Drawing for the job (mm, zero at the part's lowest x, y, z). Coordinates: 2 decimals unless noted, no trailing zeros. Write each loop counter-clockwise with the first axis right and the second up, starting at its lowest first coordinate (ties: lowest second). Pieces come first, ordered by that corner, then holes.
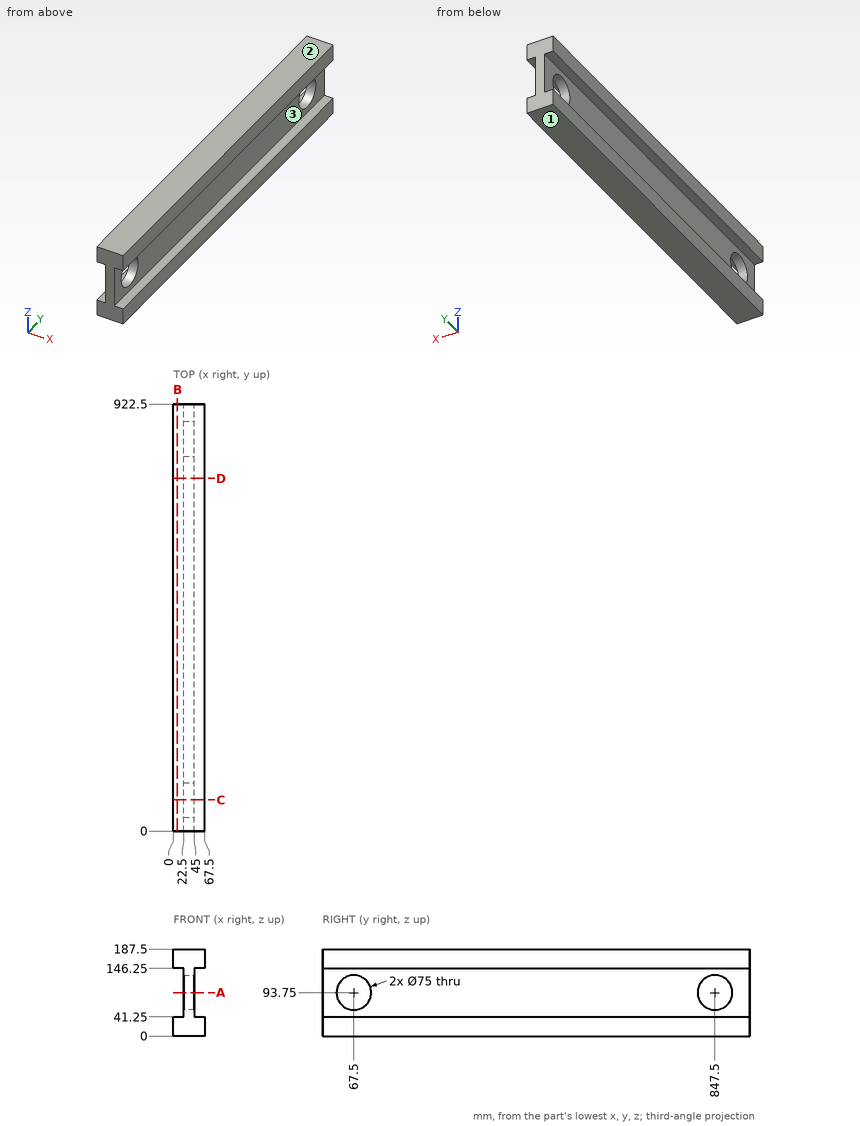
Item 1: Wall check: line 1 along Y through (x, z) = (38, 93.75); line 2 along Z through (x, y) = (3, 686.5); line 3 along Y through (x, z) = (27, 59.5). Give the ranges that are in metal, low to high.
Item 2: Two-plate mould, pull along Z, no slides. Class the marked faces 1, 2 and 3: +Z half, -Z half, draft (parallel to the pull), parting line (faces both ways), or undercut.
Item 3: Saw through at B-B, the plane x = 9. Write the cut outline in (y, z).
Item 4: Saw through at C-C, the plane y = 67.5. Write the cut outline in (x, z).
Item 5: Saw through at A-A, the plane z = 93.75. Write the cut outline in (x, y), and give its area (3 significant figures).
Item 6: Flat gauge pins, fed straight in: pin 1 Ø6 at (y, z) = (346, 87) entering from -X; pin 2 Ø12 at (y, z) = (763.5, 57.5) entering from +X. Where does each tip first touch, or does it go through?
Item 7: Saw through at D-D, the plane y = 762. Write the cut outline in (x, z).
Working result:
1. line 1: y = 0 to 30, 105 to 810, 885 to 922.5
1. line 2: z = 0 to 41.25, 146.25 to 187.5
1. line 3: y = 0 to 52.23, 82.77 to 832.23, 862.77 to 922.5
2. face 1: -Z half
2. face 2: +Z half
2. face 3: undercut
3. outline: (0, 0) - (922.5, 0) - (922.5, 41.25) - (0, 41.25) - close; (0, 146.25) - (922.5, 146.25) - (922.5, 187.5) - (0, 187.5) - close
4. outline: (0, 0) - (67.5, 0) - (67.5, 41.25) - (45, 41.25) - (45, 56.25) - (22.5, 56.25) - (22.5, 41.25) - (0, 41.25) - close; (0, 146.25) - (22.5, 146.25) - (22.5, 131.25) - (45, 131.25) - (45, 146.25) - (67.5, 146.25) - (67.5, 187.5) - (0, 187.5) - close
5. outline: (22.5, 0) - (45, 0) - (45, 30) - (22.5, 30) - close; (22.5, 105) - (45, 105) - (45, 810) - (22.5, 810) - close; (22.5, 885) - (45, 885) - (45, 922.5) - (22.5, 922.5) - close
5. area: 17,400 mm2
6. pin 1: stops at x = 22.5
6. pin 2: stops at x = 45
7. outline: (0, 0) - (67.5, 0) - (67.5, 41.25) - (45, 41.25) - (45, 146.25) - (67.5, 146.25) - (67.5, 187.5) - (0, 187.5) - (0, 146.25) - (22.5, 146.25) - (22.5, 41.25) - (0, 41.25) - close
